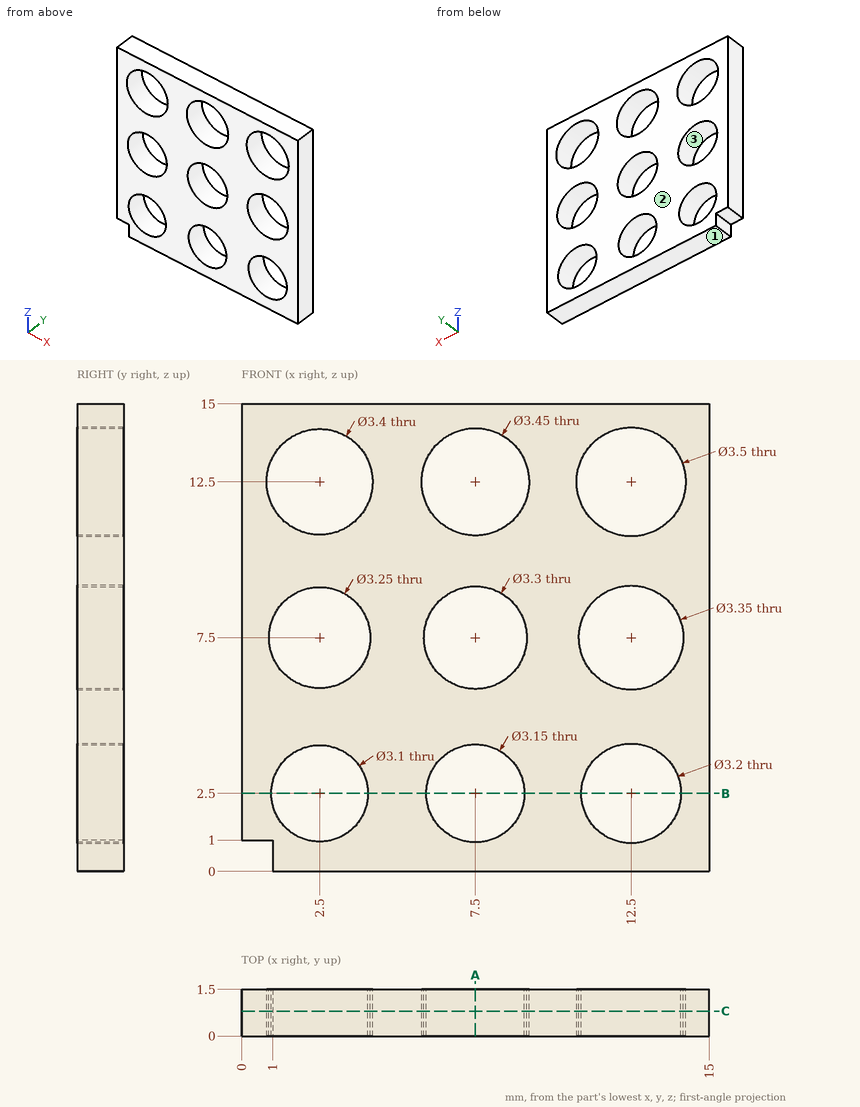
Check sheet for the drawn part. Datum: minimum x, y, z corner. Units: mm. Give positions to 0.01 mm unless a question says otherwise; leave off trailing zeros. Write each loop counter-clockwise with the first axis right and the second up, starting at its lowest first coordinate (ties: lowest second). Pieces come first, ordered by that corner, then holes.
(1) Cross-section at C-C (y = 0.8). State how many separate pieces and enclosed holes the cut face has, plus the area to 3 significant figures.
(2) Gauge pin test, flat ends, axial feed: pin 1 (1.9 mm diameter, centred on x = 12.5, z = 2.5, fed in from +Y); pin 2 (0.5 mm diameter, centred on x = 0.5, y = 0.5, fed in from -Z); pin 3 (0.5 mm diameter, centred on y = 0.5, z = 0.5, fed in from -X). Record the tip position at first contact, or that the pin passes through.
(3) Cross-section at A-A (x = 7.5). Enter the section's corners in (y, z) (3 decimals), plus the area to 3 significant figures.
(4) Material ranges on line 1 (X direction, y = 0.6, z = 7.5) (3 decimals); line 2 (X direction, y = 0.6, z = 12.5) (3 decimals); line 3 (Z direction, x = 7, y = 1.3), recorded low to high.
(5) Cross-section at B-B (z = 2.5). Enter the section's corners in (x, y) (3 decimals).
(6) Mould release check, pull along Z, two halves, no side actions. Record for the marked faces 1, 2 and 3: +Z half, -Z half, draft (parallel to the pull), parting line (faces both ways), or undercut.
Worked out:
1. separate pieces: 1
1. enclosed holes: 9
1. area: 147 mm2
2. pin 1: passes through
2. pin 2: stops at z = 1
2. pin 3: stops at x = 1
3. outline: (0, 0) - (1.5, 0) - (1.5, 0.925) - (0, 0.925) - close; (0, 4.075) - (1.5, 4.075) - (1.5, 5.85) - (0, 5.85) - close; (0, 9.15) - (1.5, 9.15) - (1.5, 10.775) - (0, 10.775) - close; (0, 14.225) - (1.5, 14.225) - (1.5, 15) - (0, 15) - close
3. area: 7.65 mm2
4. line 1: x = 0 to 0.875, 4.125 to 5.85, 9.15 to 10.825, 14.175 to 15
4. line 2: x = 0 to 0.8, 4.2 to 5.775, 9.225 to 10.75, 14.25 to 15
4. line 3: z = 0 to 1.01, 3.99 to 5.93, 9.07 to 10.85, 14.15 to 15
5. outline: (0, 0) - (0.95, 0) - (0.95, 1.5) - (0, 1.5) - close; (4.05, 0) - (5.925, 0) - (5.925, 1.5) - (4.05, 1.5) - close; (9.075, 0) - (10.9, 0) - (10.9, 1.5) - (9.075, 1.5) - close; (14.1, 0) - (15, 0) - (15, 1.5) - (14.1, 1.5) - close
6. face 1: -Z half
6. face 2: draft
6. face 3: undercut
